Work out the finished part from the listing and answer in its coordinate system (mm). Face numbers are marked on the shaded views. A direction names the side the tool comes from. Coordinates: 2 decimals unless noted, no trailing zeros. Loops run counter-clockwise (first coordinate to the right, second up) from the corner with the lowest first, then second, coordinate; pieces in that order, holes last. Notation, with made-up numbers: (33, 6) -> (47, 6) arc R27 ccw to (47, 38) -> close; hole circle Ø6 at (-10, -27). An arc over 180 degrees is marked (long way). One line per question, with ' | ' between items.
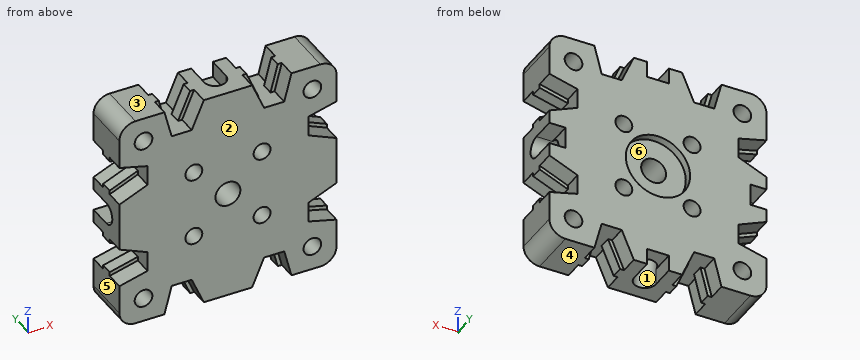
```python
from build123d import *

# Parameters (mm, degrees)
SKETCH_3_W                      = 27
SKETCH_3_H                      = 27
EXTRUDE_1_DEPTH                 = 3
FILLET_1_R                      = 2
SKETCH_4_R                      = 1.1
CUT_EXTRUDE_1_DEPTH             = 6
SKETCH_5_R                      = 1.55
CUT_EXTRUDE_2_DEPTH             = 6
SKETCH_6_R                      = 1.05
CUT_EXTRUDE_3_DEPTH             = 6
PATTERN_CIRCULAR_1_COUNT        = 4
SKETCH_7_R                      = 4
CUT_EXTRUDE_4_DEPTH             = 1
CUT_EXTRUDE_8_DEPTH             = 21.012496096
PATTERN_CIRCULAR_2_COUNT        = 4
PATTERN_CIRCULAR_2_COPY_1_DEPTH = 21.012496096
PATTERN_CIRCULAR_2_COPY_2_DEPTH = 21.012496096
PATTERN_CIRCULAR_2_COPY_3_DEPTH = 21.012496096
SKETCH_12_R                     = 1.35
CUT_EXTRUDE_9_DEPTH             = 8
PATTERN_CIRCULAR_3_COUNT        = 4
EXTRUDE_2_DEPTH                 = 0.75
PATTERN_CIRCULAR_4_COUNT        = 4
PATTERN_CIRCULAR_4_COPY_1_DEPTH = 0.75
PATTERN_CIRCULAR_4_COPY_2_DEPTH = 0.75
PATTERN_CIRCULAR_4_COPY_3_DEPTH = 0.75
SKETCH_22_W                     = 2.7
SKETCH_22_H                     = 3
CUT_EXTRUDE_15_DEPTH            = 2
PATTERN_CIRCULAR_11_COUNT       = 4


with BuildPart() as part:
    # ｽｹｯﾁ3 → ﾎﾞｽ - 押し出し1 (new, symmetric)
    with BuildSketch(Plane(origin=(0, 0, 0), x_dir=(1, 0, 0), z_dir=(0, 1, 0))):
        Rectangle(SKETCH_3_W, SKETCH_3_H)
    extrude(amount=EXTRUDE_1_DEPTH, both=True)

    # ﾌｨﾚｯﾄ1
    fillet_1_edges = [part.edges().sort_by_distance(p)[0] for p in [
        (13.5, 0, 13.5),
        (-13.5, 0, 13.5),
        (-13.5, 0, -13.5),
        (13.5, 0, -13.5),
    ]]
    fillet(fillet_1_edges, radius=FILLET_1_R)

    # ｽｹｯﾁ4 → ｶｯﾄ - 押し出し1 (cut)
    with BuildSketch(Plane(origin=(0, 3, 0), x_dir=(1, 0, 0), z_dir=(0, 1, 0))):
        with Locations(Location((-10.5, 10.5, 0), (0, 0, 270))):
            Circle(SKETCH_4_R)
        with Locations(Location((10.5, 10.5, 0), (0, 0, 270))):
            Circle(SKETCH_4_R)
        with Locations(Location((-10.5, -10.5, 0), (0, 0, 270))):
            Circle(SKETCH_4_R)
        with Locations(Location((10.5, -10.5, 0), (0, 0, 270))):
            Circle(SKETCH_4_R)
    extrude(amount=-CUT_EXTRUDE_1_DEPTH, mode=Mode.SUBTRACT)

    # ｽｹｯﾁ5 → ｶｯﾄ - 押し出し2 (cut)
    with BuildSketch(Plane(origin=(0, 3, 0), x_dir=(1, 0, 0), z_dir=(0, 1, 0))):
        with Locations(Location((0, 0, 0), (0, 0, 270))):
            Circle(SKETCH_5_R)
    extrude(amount=-CUT_EXTRUDE_2_DEPTH, mode=Mode.SUBTRACT)

    # ｽｹｯﾁ6 → ｶｯﾄ - 押し出し3 (cut)
    with BuildSketch(Plane(origin=(0, 3, 0), x_dir=(1, 0, 0), z_dir=(0, 1, 0))):
        with Locations(Location((4.242640687, 4.242640687, 0), (0, 0, 270))):
            Circle(SKETCH_6_R)
    cut_extrude_3 = extrude(amount=-CUT_EXTRUDE_3_DEPTH, mode=Mode.SUBTRACT)

    # 円形ﾊﾟﾀｰﾝ1: ｶｯﾄ - 押し出し3 ×4 about axis
    pattern_circular_1_axis = Axis((0, 0, 0), (0, 1, 0))
    for i in range(1, PATTERN_CIRCULAR_1_COUNT):
        add(cut_extrude_3.rotate(pattern_circular_1_axis, i * 360 / PATTERN_CIRCULAR_1_COUNT), mode=Mode.SUBTRACT)

    # ｽｹｯﾁ7 → ｶｯﾄ - 押し出し4 (cut)
    with BuildSketch(Plane(origin=(0, 3, 0), x_dir=(1, 0, 0), z_dir=(0, 1, 0))):
        with Locations(Location((0, 0, 0), (0, 0, 270))):
            Circle(SKETCH_7_R)
    extrude(amount=-CUT_EXTRUDE_4_DEPTH, mode=Mode.SUBTRACT)

    # ｽｹｯﾁ11 → ｶｯﾄ - 押し出し8 (cut, symmetric)
    with BuildSketch(Plane(origin=(0, 3, 0), x_dir=(1, 0, 0), z_dir=(0, 1, 0))):
        Polygon((-28.082033535, 86.024744916), (3, 13.5), (4.5, 10), (7, 10), (7.9, 13.5), (27.55047658, 89.918520033), (16.532211377, 247.342544779), (-39.100298738, 243.448769662), align=None)
    cut_extrude_8 = extrude(amount=CUT_EXTRUDE_8_DEPTH, both=True, mode=Mode.SUBTRACT)

    # ﾐﾗｰ1: ｶｯﾄ - 押し出し8 across plane
    add(cut_extrude_8.mirror(Plane(origin=(0, 0, 0), x_dir=(0, 0, 1), z_dir=(1, 0, 0))), mode=Mode.SUBTRACT)

    # 円形ﾊﾟﾀｰﾝ2: ｶｯﾄ - 押し出し8 ×4 about axis
    pattern_circular_2_axis = Axis((0, 0, 0), (0, 1, 0))
    for i in range(1, PATTERN_CIRCULAR_2_COUNT):
        add(cut_extrude_8.rotate(pattern_circular_2_axis, i * 360 / PATTERN_CIRCULAR_2_COUNT), mode=Mode.SUBTRACT)

    # 円形ﾊﾟﾀｰﾝ2 copy 1 sketch → 円形ﾊﾟﾀｰﾝ2 copy 1 (cut, symmetric)
    with BuildSketch(Plane.ZX.offset(3)):
        Polygon((-28.082033535, -86.024744916), (3, -13.5), (4.5, -10), (7, -10), (7.9, -13.5), (27.55047658, -89.918520033), (16.532211377, -247.342544779), (-39.100298738, -243.448769662), align=None)
    extrude(amount=PATTERN_CIRCULAR_2_COPY_1_DEPTH, both=True, mode=Mode.SUBTRACT)

    # 円形ﾊﾟﾀｰﾝ2 copy 2 sketch → 円形ﾊﾟﾀｰﾝ2 copy 2 (cut, symmetric)
    with BuildSketch(Plane(origin=(0, 3, 0), x_dir=(1, 0, 0), z_dir=(0, 1, 0))):
        Polygon((-28.082033535, -86.024744916), (3, -13.5), (4.5, -10), (7, -10), (7.9, -13.5), (27.55047658, -89.918520033), (16.532211377, -247.342544779), (-39.100298738, -243.448769662), align=None)
    extrude(amount=PATTERN_CIRCULAR_2_COPY_2_DEPTH, both=True, mode=Mode.SUBTRACT)

    # 円形ﾊﾟﾀｰﾝ2 copy 3 sketch → 円形ﾊﾟﾀｰﾝ2 copy 3 (cut, symmetric)
    with BuildSketch(Plane(origin=(0, 3, 0), x_dir=(0, 0, -1), z_dir=(0, 1, 0))):
        Polygon((-28.082033535, -86.024744916), (3, -13.5), (4.5, -10), (7, -10), (7.9, -13.5), (27.55047658, -89.918520033), (16.532211377, -247.342544779), (-39.100298738, -243.448769662), align=None)
    extrude(amount=PATTERN_CIRCULAR_2_COPY_3_DEPTH, both=True, mode=Mode.SUBTRACT)

    # ｽｹｯﾁ12 → ｶｯﾄ - 押し出し9 (cut)
    with BuildSketch(Plane.XY.offset(13.5)):
        Circle(SKETCH_12_R)
    cut_extrude_9 = extrude(amount=-CUT_EXTRUDE_9_DEPTH, mode=Mode.SUBTRACT)

    # 円形ﾊﾟﾀｰﾝ3: ｶｯﾄ - 押し出し9 ×4 about axis
    pattern_circular_3_axis = Axis((0, 0, 0), (0, 1, 0))
    for i in range(1, PATTERN_CIRCULAR_3_COUNT):
        add(cut_extrude_9.rotate(pattern_circular_3_axis, i * 360 / PATTERN_CIRCULAR_3_COUNT), mode=Mode.SUBTRACT)

    # ｽｹｯﾁ13 → ﾎﾞｽ - 押し出し2 (add, symmetric)
    with BuildSketch(Plane(origin=(0, 0, 0), x_dir=(1, 0, 0), z_dir=(0, 1, 0))):
        Polygon((7.9, 13.5), (7, 10), (6.5, 10), (7.4, 13.5), align=None)
        Polygon((3, 13.5), (3.5, 13.5), (5, 10), (4.5, 10), align=None)
    extrude_2 = extrude(amount=EXTRUDE_2_DEPTH, both=True)

    # ﾐﾗｰ2: ﾎﾞｽ - 押し出し2 across plane
    add(extrude_2.mirror(Plane(origin=(0, 0, 0), x_dir=(0, 0, 1), z_dir=(1, 0, 0))))

    # 円形ﾊﾟﾀｰﾝ4: ﾎﾞｽ - 押し出し2 ×4 about axis
    pattern_circular_4_axis = Axis((0, 0, 0), (0, 1, 0))
    for i in range(1, PATTERN_CIRCULAR_4_COUNT):
        add(extrude_2.rotate(pattern_circular_4_axis, i * 360 / PATTERN_CIRCULAR_4_COUNT))

    # 円形ﾊﾟﾀｰﾝ4 copy 1 sketch → 円形ﾊﾟﾀｰﾝ4 copy 1 (add, symmetric)
    with BuildSketch(Plane.ZX):
        Polygon((7.9, -13.5), (7, -10), (6.5, -10), (7.4, -13.5), align=None)
        Polygon((3, -13.5), (3.5, -13.5), (5, -10), (4.5, -10), align=None)
    extrude(amount=PATTERN_CIRCULAR_4_COPY_1_DEPTH, both=True)

    # 円形ﾊﾟﾀｰﾝ4 copy 2 sketch → 円形ﾊﾟﾀｰﾝ4 copy 2 (add, symmetric)
    with BuildSketch(Plane(origin=(0, 0, 0), x_dir=(1, 0, 0), z_dir=(0, 1, 0))):
        Polygon((7.9, -13.5), (7, -10), (6.5, -10), (7.4, -13.5), align=None)
        Polygon((3, -13.5), (3.5, -13.5), (5, -10), (4.5, -10), align=None)
    extrude(amount=PATTERN_CIRCULAR_4_COPY_2_DEPTH, both=True)

    # 円形ﾊﾟﾀｰﾝ4 copy 3 sketch → 円形ﾊﾟﾀｰﾝ4 copy 3 (add, symmetric)
    with BuildSketch(Plane(origin=(0, 0, 0), x_dir=(0, 0, -1), z_dir=(0, 1, 0))):
        Polygon((7.9, -13.5), (7, -10), (6.5, -10), (7.4, -13.5), align=None)
        Polygon((3, -13.5), (3.5, -13.5), (5, -10), (4.5, -10), align=None)
    extrude(amount=PATTERN_CIRCULAR_4_COPY_3_DEPTH, both=True)

    # ｽｹｯﾁ22 → ｶｯﾄ - 押し出し15 (cut)
    with BuildSketch(Plane.XY.offset(13.5)):
        with Locations((0, 1.5)):
            Rectangle(SKETCH_22_W, SKETCH_22_H)
    cut_extrude_15 = extrude(amount=-CUT_EXTRUDE_15_DEPTH, mode=Mode.SUBTRACT)

    # 円形ﾊﾟﾀｰﾝ11: ｶｯﾄ - 押し出し15 ×4 about axis
    pattern_circular_11_axis = Axis((0, 0, 0), (0, 1, 0))
    for i in range(1, PATTERN_CIRCULAR_11_COUNT):
        add(cut_extrude_15.rotate(pattern_circular_11_axis, i * 360 / PATTERN_CIRCULAR_11_COUNT), mode=Mode.SUBTRACT)


solid = part.part
```
1) Find section C-C (x = -10.5). State how many separate pieces and enclosed holes the cut face has, plus the area to 3 significant figures.
Check values:
separate pieces: 5 | enclosed holes: 1 | area: 98.8 mm^2
2) Find the intervals of material crossed by line 1 along Z through (x, y) = (-11.25, 0); line 2 along Y through (x, z) = (0, -9.25); line 3 along X through (y, z) = (-1, -12), in increasing order.
Check values:
line 1: z = -13.5 to -11.3, -9.7 to -6.82, -4.46 to -1.35, 1.35 to 4.46, 6.82 to 9.7, 11.3 to 13.5 | line 2: y = -3 to -1.35, 1.35 to 3 | line 3: x = -13.44 to -7.51, -3.64 to -0.91, 0.91 to 3.64, 7.51 to 13.44
3) Find section A-A (x = 0). Write down the section's boundary in (y, z).
Check values:
outline: (-3, -13.5) -> (-1.35, -13.5) -> (-1.35, -5.5) -> (1.35, -5.5) -> (1.35, -11.5) -> (3, -11.5) -> (3, -4) -> (2, -4) -> (2, -1.55) -> (-3, -1.55) -> close; (-3, 1.55) -> (2, 1.55) -> (2, 4) -> (3, 4) -> (3, 11.5) -> (1.35, 11.5) -> (1.35, 5.5) -> (-1.35, 5.5) -> (-1.35, 13.5) -> (-3, 13.5) -> close
4) For the marked faces 1 and 2, determine the directions among +Z, -Z, +X, -X, +Y, -Y from which every point of the face is accessible in a straight line to the end or side of a thin tool.
Check values:
face 1: -Z | face 2: +Z, -Z, +X, -X, -Y
5) The mould has two halves that part along Z. Classify the marked faces 3, 4, 5 and 6: released by +Z, released by -Z, zero draft, split by the parting line, or undercut.
Check values:
face 3: released by +Z | face 4: released by -Z | face 5: zero draft | face 6: undercut
6) Flat-ended cylindrical pins translate along their axes: pin 1 (0.6 mm diameter, centred on x = -12, y = 1.5, fed in from +Z); pin 2 (0.6 mm diameter, centred on x = -11.5, z = 4.5, fed in from +Y); pin 3 (0.6 mm diameter, centred on x = 13, y = 1, fed in from -Z). Find the tip coordinate at first contact, or state that the pin passes through.
Check values:
pin 1: stops at z = 13.49 | pin 2: stops at y = 0.75 | pin 3: stops at z = -13.1
7) Find section B-B (z = -2). Write down the section's boundary in (x, y), plus the area to 3 significant figures.
Check values:
outline: (-13.5, -3) -> (13.5, -3) -> (13.5, 3) -> (3.46, 3) -> (3.46, 2) -> (-3.46, 2) -> (-3.46, 3) -> (-13.5, 3) -> close | area: 155 mm^2
